Here's how the part is built. I have some questions about the finished solid (model axes, mm). A direction names the side the tool comes from. Coordinates: 2 decimals unless noted, no trailing zeros.
from build123d import *

# Parameters (mm, degrees)
SKETCH1_W           = 177.8
SKETCH1_H           = 355.6
BOSS_EXTRUDE1_DEPTH = 12.7
SKETCH3_R           = 2.159
CUT_EXTRUDE1_DEPTH  = 398.775677989


with BuildPart() as part:
    # Sketch1 → Boss-Extrude1 (new body)
    with BuildSketch(Plane.XY):
        with Locations((88.9, 177.8)):
            Rectangle(SKETCH1_W, SKETCH1_H)
    extrude(amount=BOSS_EXTRUDE1_DEPTH)

    # Sketch3 → Cut-Extrude1 (cut, through all)
    with BuildSketch(Plane.XY.offset(12.7)):
        with Locations((7.62, 330.2)):
            Circle(SKETCH3_R)
        with Locations((7.62, 279.4)):
            Circle(SKETCH3_R)
        with Locations(Location((7.62, 76.2, 0), (0, 0, 180))):
            Circle(SKETCH3_R)
        with Locations(Location((7.62, 25.4, 0), (0, 0, 180))):
            Circle(SKETCH3_R)
        Polygon((177.8, 332.359), (170.18, 332.359), (170.18, 333.883), (166.878, 333.883), (166.878, 332.359), (162.56, 332.359), (162.56, 328.041), (166.878, 328.041), (166.878, 326.517), (170.18, 326.517), (170.18, 328.041), (177.8, 328.041), align=None)
        Polygon((177.8, 281.559), (177.8, 277.241), (170.18, 277.241), (170.18, 275.717), (166.878, 275.717), (166.878, 277.241), (162.56, 277.241), (162.56, 281.559), (166.878, 281.559), (166.878, 283.083), (170.18, 283.083), (170.18, 281.559), align=None)
        Polygon((177.8, 78.359), (170.18, 78.359), (170.18, 79.883), (166.878, 79.883), (166.878, 78.359), (162.56, 78.359), (162.56, 74.041), (166.878, 74.041), (166.878, 72.517), (170.18, 72.517), (170.18, 74.041), (177.8, 74.041), align=None)
        Polygon((177.8, 27.559), (177.8, 23.241), (170.18, 23.241), (170.18, 21.717), (166.878, 21.717), (166.878, 23.241), (162.56, 23.241), (162.56, 27.559), (166.878, 27.559), (166.878, 29.083), (170.18, 29.083), (170.18, 27.559), align=None)
        Polygon((177.8, 205.359), (170.18, 205.359), (170.18, 206.883), (166.878, 206.883), (166.878, 205.359), (162.56, 205.359), (162.56, 201.041), (166.878, 201.041), (166.878, 199.517), (170.18, 199.517), (170.18, 201.041), (177.8, 201.041), align=None)
        Polygon((177.8, 154.559), (177.8, 150.241), (170.18, 150.241), (170.18, 148.717), (166.878, 148.717), (166.878, 150.241), (162.56, 150.241), (162.56, 154.559), (166.878, 154.559), (166.878, 156.083), (170.18, 156.083), (170.18, 154.559), align=None)
    extrude(amount=-CUT_EXTRUDE1_DEPTH, mode=Mode.SUBTRACT)


solid = part.part
Q1. Please list where these lines run through material, in increasing order: probe 1 along Y at (x, z) = (7.62, 6.75); probe 2 along X at (y, z) = (282.5, 7.5); probe 3 along X at (y, z) = (279.4, 3).
Q2. For faces 4 (the flat face through (174, 27.559, 6)), 5 (the flat face through (177.8, 177, 6)), which set-ups out of +Z, -Z, +X, -X, +Y, -Y let a thin tool reach every point of the face, with its end or its side?
Q3. We'd pull the mould along Y, two halves only. Please class faces 1 (the flat face through (174, 328.041, 6)), 2 (the flat face through (88, 355.6, 6)), 3 (the flat face through (177.8, 11, 6)): pulls with the +Y half, pulls with the -Y half, needs draft (parallel to the pull), parting line crosses it, or undercut.
Q4. Will this pin go through, and if not, where does the flat tip stop? P1, Ø3.5, axis at x = 168.5, z = 3.5, coming from the -Y side.
Check values:
1. probe 1: y = 0 to 23.24, 27.56 to 74.04, 78.36 to 277.24, 281.56 to 328.04, 332.36 to 355.6
1. probe 2: x = 0 to 166.88, 170.18 to 177.8
1. probe 3: x = 0 to 5.46, 9.78 to 162.56
2. face 4: +Z, -Z, +X
2. face 5: +Z, -Z, +X, +Y, -Y
3. face 1: undercut
3. face 2: pulls with the +Y half
3. face 3: needs draft
4. P1: stops at y = 0
